```python
from build123d import *

# Parameters (mm, degrees)
CUT_EXTRUDE1_DEPTH = 1.3


with BuildPart() as part:
    # Sketch1 → Revolve1 (revolve)
    with BuildSketch(Plane.XY):
        with BuildLine():
            Line((-2.86, 0), (-2.86, 2.45))
            Line((-2.86, 2.45), (-2.56, 2.75))
            Line((-2.56, 2.75), (0, 2.75))
            Line((0, 2.75), (0, 1.7))
            ThreePointArc((0, 1.7), (0.058578644, 1.558578644), (0.2, 1.5))
            Line((0.2, 1.5), (11.7295, 1.5))
            Line((11.7295, 1.5), (12, 1.2295))
            Line((12, 1.2295), (12, 0))
            Line((12, 0), (-2.86, 0))
        make_face()
    revolve(axis=Axis((12, 0, 0), (-1, 0, 0)))

    # Sketch2 → Cut-Extrude1 (cut)
    with BuildSketch(Plane(origin=(-2.86, 0, 0), x_dir=(0, 0, -1), z_dir=(1, 0, 0))):
        Polygon((-1.25, 0.721687836), (-1.25, -0.721687836), (0, -1.443375673), (1.25, -0.721687836), (1.25, 0.721687836), (0, 1.443375673), align=None)
    extrude(amount=CUT_EXTRUDE1_DEPTH, mode=Mode.SUBTRACT)

    # Sketch3 → Cut-Revolve1 (revolve, cut)
    with BuildSketch(Plane.XY):
        Polygon((-1.56, 0), (-1.56, 1.25), (-0.838312164, 0), align=None)
    revolve(axis=Axis((-0.838312164, 0, 0), (-1, 0, 0)), mode=Mode.SUBTRACT)


solid = part.part
```
Geometry: final body of the model. Coordinates: model frame, mm. A direction names the side the tool comes from. Coordinates: 2 decimals unless noted, no trailing zeros. Order: outer loops, then holes, each group sorted by start corner. A loop starts at its lowest first (then second) coordinate and runs counter-clockwise, first axis right, second up. Notation, with made-up numbers: (71.5, 19.5) -> (83.5, 19.5) arc R16 cw to (83.5, 46.5) -> close; hole circle Ø4 at (59.25, 34). An arc over 180 degrees is marked (long way). Use CSV: the item, a comma, the result in double quotes.
1) Access query for faces 1 (the cylindrical face through (6.05, -1.5, -0.07)), 2 (the flat face through (-2, 0, 1.25)), 3 (the flat face through (12, 0, 0)). Directions: +Z, -Z, +X, -X, +Y, -Y. A direction counts if a zero-diameter tool reaches every point of the face in a straight line with its end or side. Return the directions, or none.
Findings:
face 1,"+X"
face 2,"-X"
face 3,"+Z, -Z, +X, +Y, -Y"
2) Line query: line 1 (X direction, y = 1.7, z = -0.5); line 2 (X direction, y = 0.3, z = -0.6); line 3 (Y direction, x = 9, z = -0.1). Output: solid intervals per line, ascending.
Findings:
line 1,"x = -2.86 to 0"
line 2,"x = -1.23 to 12"
line 3,"y = -1.5 to 1.5"
3) Section A-A on x = 4.5. Output: boundary loops of the cut face in (y, z).
Findings:
outline,"circle Ø3 at (0, 0)"
4) Mould query, pull axis Y, two halves, no side actions, for faces 4 (the flat face through (0, 2, 0)), 5 (the flat face through (-2.219, 1.088, 0.616)), 6 (the conical face through (-0.954, -0.158, 0.121)), 7 (the cylindrical face through (-1.262, -0.596, 2.685)). Classes: +Y half, -Y half, draft (parallel to the pull), parting line (faces both ways), or undercut.
Findings:
face 4,"draft"
face 5,"undercut"
face 6,"undercut"
face 7,"parting line"
5) Pin query (flat end, axial travel): pin 1 Ø2 at (x, y) = (4, 1.5) entering from +Z; pin 2 Ø2 at (x, z) = (10.5, -1) entering from -Y; pin 3 Ø3 at (x, z) = (9, -0.5) entering from +Y. Return the tip coordinate at first contact, or that it passes through.
Findings:
pin 1,"stops at z = 1.41"
pin 2,"stops at y = -1.5"
pin 3,"stops at y = 1.5"
